CAD build for the part. Positions are in the model's coordinates, mm. Face numbers are marked on the shaded views. A direction names the side the tool comes from. Give positions to 0.01 mm unless a question says otherwise; leave off trailing zeros. Order: outer loops, then holes, each group sorted by start corner. A loop starts at its lowest first (then second) coordinate and runs counter-clockwise, first axis right, second up.
Item 1: Two-plate mould, pull along X, no slides. Class the marked faces 1, 2 and 3: released by +X, released by -X, zero draft, split by the parting line, or undercut.
Item 2: Band-saw the part on A-A on x = -13.5. Give the cut face in (y, z).
Item 3: Wall check: L1, parallel to Z at x = -14.5, y = 6.75; L2, parallel to Y at x = -26, z = 3.95; L3, parallel to Y at x = -20, z = 4.4. Give the ranges that are in metal, low to high.
Item 4: Flat gauge pins, fed straight in: P1, Ø1.2, axis at x = 0, y = 0, coming from the +Z side; P2, Ø2, axis at y = 3.5, z = 3, coming from the -X side. Where does each tip first touch, or does it go through?
Item 5: Band-saw the part on D-D on y = 3. Give the cut face in (x, z), plus the area to 3 significant figures.
Item 6: Band-saw the part on B-B on z = 0.75. Give the cut face in (x, y) (1 decimal).
Item 7: Band-saw the part on C-C on x = -20. Give the cut face in (y, z), plus the area to 3 significant figures.
Item 8: Which spindle directions (+Z, -Z, +X, -X, +Y, -Y) get a long thin tool onto all of the face, cutting with end or side? Do the marked faces 4 and 5. Say none if no direction does.
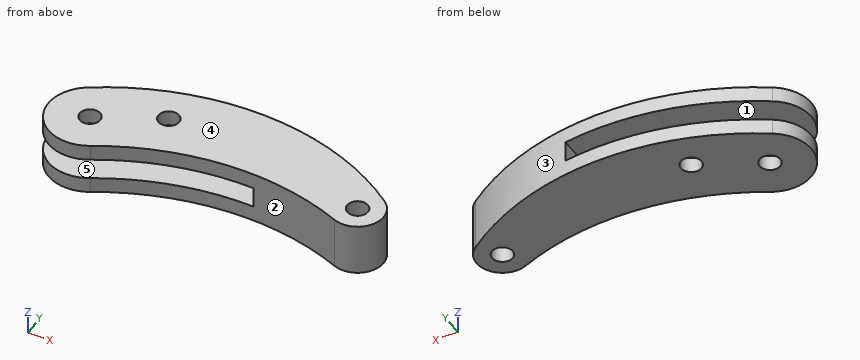
Autodesk Inventor part; units mm, degrees
ref_plane "Work Plane1" through (0, 0, 0.75) normal (0, 0, 1) x (1, 0, 0)
ref_plane "YZ Plane" through (0, 0, 0) normal (1, 0, 0) x (0, 1, 0)
ref_plane "XZ Plane" through (0, 0, 0) normal (0, 1, 0) x (-1, 0, 0)
sketch "Sketch1" plane through (0, 0, 0) normal (0, 0, 1) x (1, 0, 0)
  circle A0 centre (0, 0) radius 1
  circle A1 centre (-20, 3) radius 1
  circle A2 centre (-26, 0) radius 1
  arc A3 (-0.9923, -2.2946) -> (1.5226, 1.9828) centre (0, 0) ccw
  arc A4 (-28.125, 3.3889) -> (-24.0417, -3.4878) centre (-26, 0) ccw
  arc A5 (1.5226, 1.9828) -> (-28.125, 3.3889) centre (-14.3125, -18.6387) ccw
  arc A6 (-0.9923, -2.2946) -> (-24.0417, -3.4878) centre (-11.3125, -26.1587) ccw
  dimension "d50" = 2
  dimension "d51" = 3
  dimension "d52" = 20
  dimension "d53" = 6
  dimension "d55" = 2.5
  dimension "d56" = 4
  dimension "d57" = 26
  dimension "d58" = 26
extrude "Extrusion1" add sketch "Sketch1" along normal blind 5
sketch "Sketch3" plane through (0, 0, 0) normal (0, 1, 0) x (-1, 0, 0)
  line L0 (10, 1.5) -> (45.3794, 1.5)
  line L1 (45.3794, 1.5) -> (45.3794, 3.5)
  line L2 (45.3794, 3.5) -> (10, 3.5)
  line L3 (10, 3.5) -> (10, 1.5)
  line L4 (-0.0755, 0) -> (-0.0755, 5)
  point P0 (0, 0)
  dimension "d34" = 1.5
  dimension "d35" = 10
  dimension "d36" = 2
extrude "Extrusion3" cut sketch "Sketch3" along normal through all both and the other way through all
properties part number "legA_mini"
The answers:
1. face 1: zero draft
1. face 2: undercut
1. face 3: split by the parting line
2. outline: (-0.25, 0) - (7.35, 0) - (7.35, 1.5) - (-0.25, 1.5) - close; (-0.25, 3.5) - (7.35, 3.5) - (7.35, 5) - (-0.25, 5) - close
3. L1: z = 0 to 1.5, 3.5 to 5
3. L2: y = -4 to -1, 1 to 4.59
3. L3: y = -1.65 to 2, 4 to 6.73
4. P1: passes through
4. P2: stops at x = -29.01
5. outline: (-28.65, 0) - (-21, 0) - (-21, 1.5) - (-28.65, 1.5) - close; (-28.65, 3.5) - (-21, 3.5) - (-21, 5) - (-28.65, 5) - close; (-19, 0) - (0.1, 0) - (0.1, 5) - (-19, 5) - (-19, 3.5) - (-10, 3.5) - (-10, 1.5) - (-19, 1.5) - close
5. area: 100 mm2
6. outline: (-28.1, 3.4) arc R4 ccw to (-24, -3.5) arc R26 cw to (-1, -2.3) arc R2.5 ccw to (1.5, 2) arc R26 ccw to start; hole circle Ø2 at (-26, 0); hole circle Ø2 at (-20, 3); hole circle Ø2 at (0, 0)
7. outline: (-1.65, 0) - (2, 0) - (2, 1.5) - (-1.65, 1.5) - close; (-1.65, 3.5) - (2, 3.5) - (2, 5) - (-1.65, 5) - close; (4, 0) - (6.73, 0) - (6.73, 1.5) - (4, 1.5) - close; (4, 3.5) - (6.73, 3.5) - (6.73, 5) - (4, 5) - close
7. area: 19.2 mm2
8. face 4: +Z, +X, -X, +Y, -Y
8. face 5: -X, +Y, -Y
